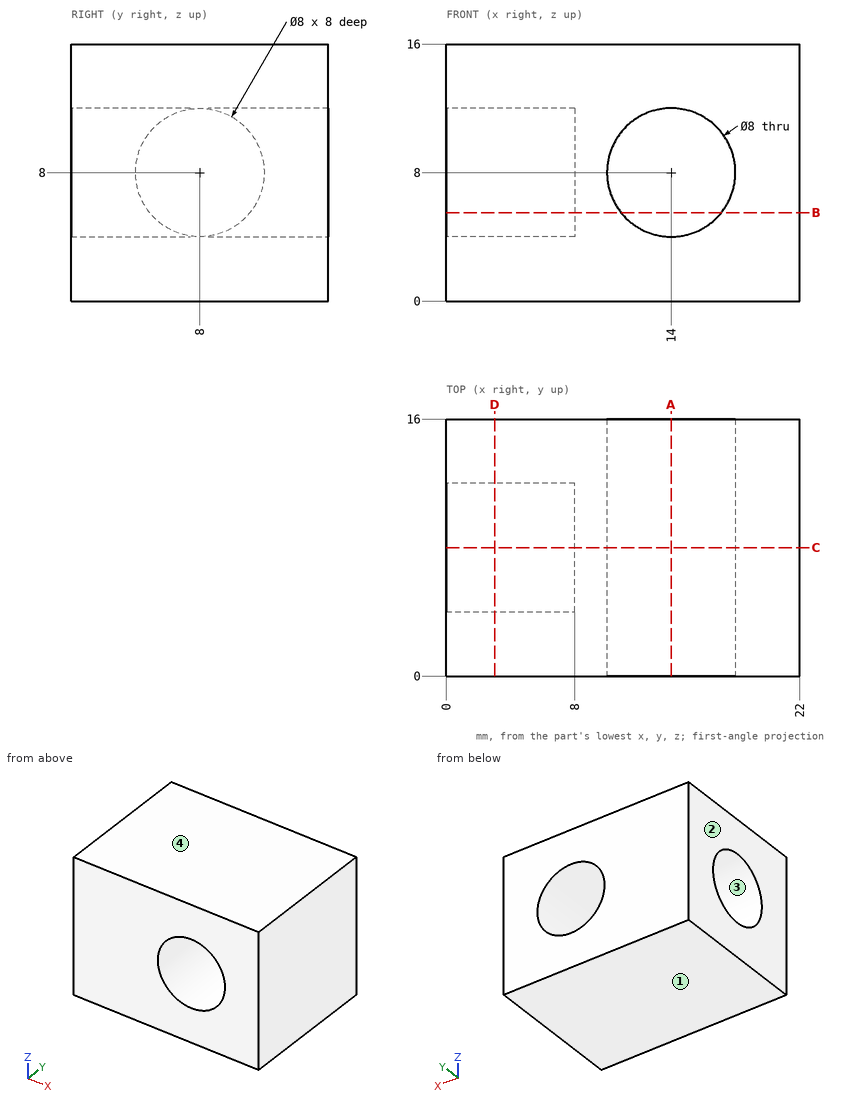
Part print with two shaded views. Sizes in mm from the minimum x, y, z corner. Coordinates: 2 decimals unless noted, no trailing zeros. Write each loop counter-clockwise with the first axis right and the second up, starting at its lowest first coordinate (ties: lowest second). Pieces come first, ordered by that corner, then holes. Notation, with made-up numbers: M 37,18 L 52,18 A18 cw 52,27 Z; hole C -1.75,81 d4. An arc over 180 degrees is marked long. Return JSON: item names as keys, results as strings.
Item 1: Probe line 1 (X direction, y = 5.75, z = 8); line 2 (Z direction, x = 3.5, y = 8); line 3 (X direction, y = 6.75, z = 10.5). List the from-to ranges inside material, lowest first. Write a range as from..to.
Findings below:
{"line 1": "x = 8..10, 18..22", "line 2": "z = 0..4, 12..16", "line 3": "x = 8..10.88, 17.12..22"}
Item 2: Slice it at B-B, the plane z = 5.5. Write the cut outline in (x, y).
Findings below:
{"outline": "M 0,0 L 10.88,0 L 10.88,16 L 0,16 L 0,11.12 L 8,11.12 L 8,4.88 L 0,4.88 Z; M 17.12,0 L 22,0 L 22,16 L 17.12,16 Z"}
Item 3: Slice it at D-D, the plane x = 3. Write the cut outline in (y, z), and give its area (3 significant figures).
Findings below:
{"outline": "M 0,0 L 16,0 L 16,16 L 0,16 Z; hole C 8,8 d8", "area": "206 mm2"}
Item 4: Two-plate mould, pull along Z, no slides. Class the marked faces 1, 2, 3 and 4: +Z half, -Z half, draft (parallel to the pull), parting line (faces both ways), or undercut.
Findings below:
{"face 1": "-Z half", "face 2": "draft", "face 3": "undercut", "face 4": "+Z half"}
Item 5: Drop a flat-ended pin along its axis: pin 1 Ø4 at (y, z) = (6.5, 7) entering from -X. Give the stop position or say it passes through.
Findings below:
{"pin 1": "stops at x = 8"}
Item 6: Slice it at C-C, the plane y = 8. Write the cut outline in (x, z).
Findings below:
{"outline": "M 0,0 L 22,0 L 22,16 L 0,16 L 0,12 L 8,12 L 8,4 L 0,4 Z; hole C 14,8 d8"}
Item 7: Slice it at A-A, the plane x = 14. Write the cut outline in (y, z).
Findings below:
{"outline": "M 0,0 L 16,0 L 16,4 L 0,4 Z; M 0,12 L 16,12 L 16,16 L 0,16 Z"}
